Here's the drawing with two shaded views (mm, measured from the low corner). I have some questions. A direction names the side the tool comes from. Coordinates: 2 decimals unless noted, no trailing zeros. Write each loop counter-clockwise with the first axis right and the second up, starting at its lowest first coordinate (ties: lowest second). Pieces come first, ordered by that corner, then holes. Notation, with made-up numbers: M 41.25,-4.75 L 99.25,-4.75 A21 ccw 99.25,7.25 Z; hole C 70,43.5 d6. An arc over 180 degrees is marked long. Answer as CSV lines item,"result". Start each with the question number.
Item 1: If I drill on line 1 along Z through (x, y) = (1.5, 1); line 2 along Y through (x, z) = (1.4, 1.5); line 3 along Z through (x, y) = (2.2, 2.9), over which ranges is the centre line in solid material (lowest first)? Write a range as [from, to].
Item 2: Suppose I cut it at B-B, the plane x = 2.2. Write out the boundary of the cut face in (y, z).
Item 3: Suppose I cut it at D-D, the plane z = 7.5. Write out the boundary of the cut face in (x, y).
Item 4: Suppose I cut it at C-C, the plane y = 1.65. Write out the boundary of the cut face in (x, z), and give its area (3 significant figures).
Item 5: We'd pull the mould along Y, two halves only. Please class the marked faces 1, 2 and 3: +Y half, -Y half, draft (parallel to the pull), parting line (faces both ways), or undercut.
Item 6: Suppose I cut it at A-A, the plane z = 1.25. Write out the boundary of the cut face in (x, y).
Item 7: On a 3-axis mill with a long thin cutter (end or side, diameter ignored), from which of +Z, -Z, +X, -X, +Y, -Y can I reach the whole of each face in a straight line? I mean the marked faces 4 and 5. Say none if no direction works.
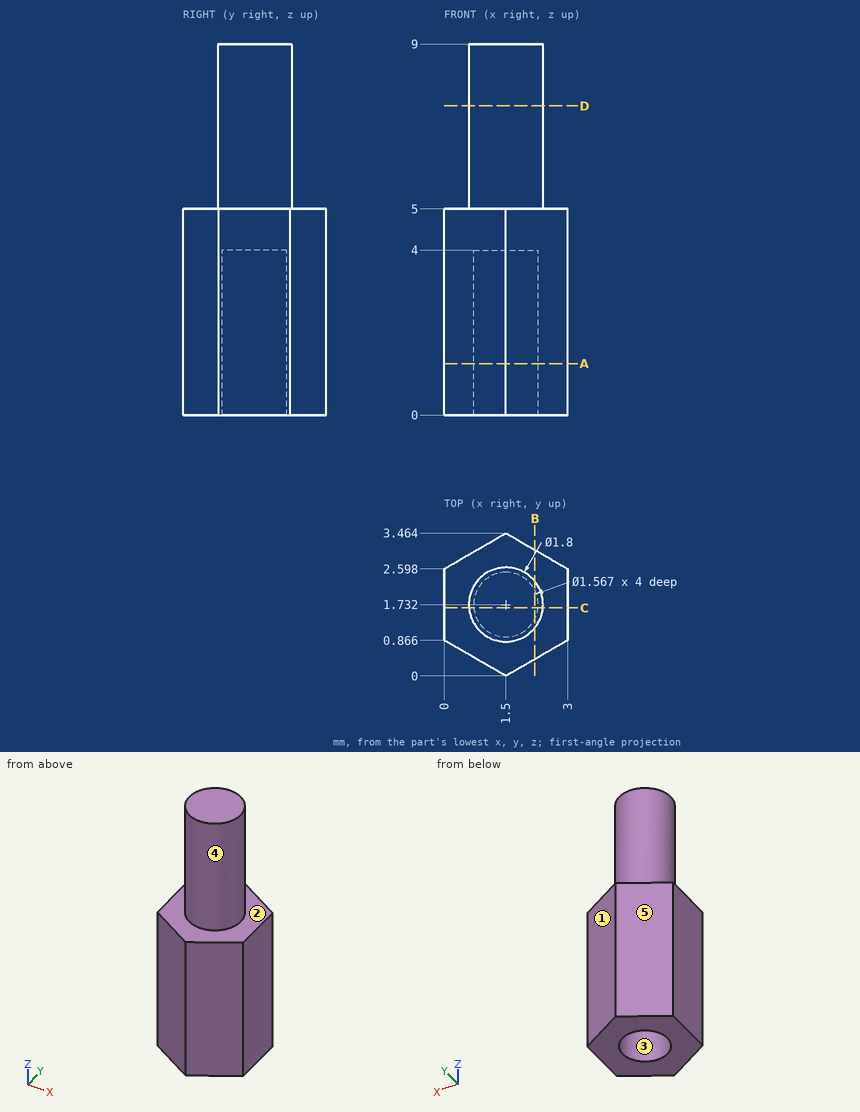
Ans:
1,line 1,"z = [4, 9]"
1,line 2,"y = [0.06, 0.95], [2.51, 3.41]"
1,line 3,"z = [0, 5]"
2,outline,"M 0.4,0 L 1.38,0 L 1.38,4 L 2.08,4 L 2.08,0 L 3.06,0 L 3.06,5 L 2.3,5 L 2.3,9 L 1.17,9 L 1.17,5 L 0.4,5 Z"
3,outline,"C 1.5,1.73 d1.8"
4,outline,"M 0,0 L 0.72,0 L 0.72,4 L 2.28,4 L 2.28,0 L 3,0 L 3,5 L 2.4,5 L 2.4,9 L 0.6,9 L 0.6,5 L 0,5 Z"
4,area,"15.9 mm^2"
5,face 1,"+Y half"
5,face 2,"draft"
5,face 3,"undercut"
6,outline,"M 0,0.87 L 1.5,0 L 3,0.87 L 3,2.6 L 1.5,3.46 L 0,2.6 Z; hole C 1.5,1.73 d1.57"
7,face 4,"+Z"
7,face 5,"+Z, -Z, -X, +Y"
